The listing builds one solid part. Answer for the finished solid, in the listing's coordinates (mm). Round coordinates to 2 decimals unless told otherwise and drop trailing zeros. Write each loop counter-clockwise with the first axis right and the second up, starting at its lowest first coordinate (ties: lowest second). Pieces come first, ordered by that corner, then holes. Notation, with made-up numbers: M 43,-1.75 L 85,-1.75 A31 ccw 85,30.25 Z; hole C 29.5,-26 d2. An arc over 180 degrees is marked long. One line per item, written item: value. Start each with the question number.
(1) Section B-B (x = 0) is taken. Determine the outline of the cut face in (y, z), plus the area to 3 significant figures.
(2) Given P1, Ø8, axis at x = 68.5, y = 27, coming from the +Z side; P2, Ø3, axis at x = 14, y = 25.5, coming from the +Z side; P3, Ø5, axis at x = -91.5, y = 15, coming from the -Z side, each flat-ended and moving along its own axis, determine where each tip first touches the part or whether it passes through.
(3) Section D-D (x = -73.5) is taken. Determine the outline of the cut face in (y, z).
(4) Section A-A (z = 0) is taken. Determine the outline of the cut face in (x, y), plus the area to 3 significant figures.
(5) Section C-C (y = 24.25) is taken. Determine the outline of the cut face in (x, z).
(6) Consider probe 1 along Z at (x, y) = (0, 18.25); probe 2 along Z at (x, y) = (11.5, 26.75); probe 3 along Z at (x, y) = (0, 8.75). Determine where each line is inside the solid, lowest interval first.
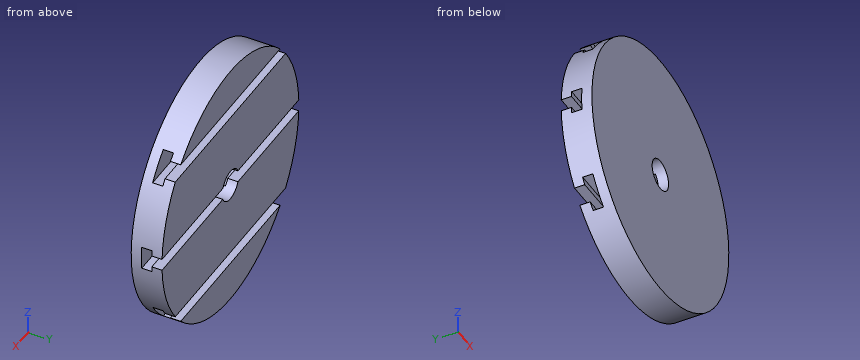
```python
from build123d import *

# Parameters (mm, degrees)
SKETCH_1_W          = 110
SKETCH_1_H          = 30
CUT_EXTRUDE_1_DEPTH = 150


with BuildPart() as part:
    # Эскиз1 → Повернуть1 (revolve)
    with BuildSketch(Plane(origin=(0, 0, 0), x_dir=(0, 0, -1), z_dir=(1, 0, 0))):
        with Locations((70, 15)):
            Rectangle(SKETCH_1_W, SKETCH_1_H)
    revolve(axis=Axis((0, -12.628115938, 0), (0, 1, 0)))

    # Эскиз2 → Вырез-Вытянуть1 (cut, symmetric)
    with BuildSketch(Plane(origin=(0, 0, 0), x_dir=(0, 0, -1), z_dir=(1, 0, 0))):
        Polygon((11.5, 10), (11.5, 20), (6, 20), (6, 30), (-6, 30), (-6, 20), (-11.5, 20), (-11.5, 10), align=None)
        Polygon((68.5, 10), (91.5, 10), (91.5, 20), (86, 20), (86, 30), (74, 30), (74, 20), (68.5, 20), align=None)
        Polygon((-91.5, 10), (-68.5, 10), (-68.5, 20), (-74, 20), (-74, 30), (-86, 30), (-86, 20), (-91.5, 20), align=None)
    extrude(amount=CUT_EXTRUDE_1_DEPTH, both=True, mode=Mode.SUBTRACT)


solid = part.part
```
Recorded:
1. outline: M 0,-125 L 30,-125 L 30,-86 L 20,-86 L 20,-91.5 L 10,-91.5 L 10,-68.5 L 20,-68.5 L 20,-74 L 30,-74 L 30,-15 L 0,-15 Z; M 0,15 L 30,15 L 30,74 L 20,74 L 20,68.5 L 10,68.5 L 10,91.5 L 20,91.5 L 20,86 L 30,86 L 30,125 L 0,125 Z
1. area: 5,900 mm2
2. P1: stops at z = 107.07
2. P2: stops at z = 124.37
2. P3: stops at z = -68.5
3. outline: M 0,-101.11 L 30,-101.11 L 30,-86 L 20,-86 L 20,-91.5 L 10,-91.5 L 10,-68.5 L 20,-68.5 L 20,-74 L 30,-74 L 30,-6 L 20,-6 L 20,-11.5 L 10,-11.5 L 10,11.5 L 20,11.5 L 20,6 L 30,6 L 30,74 L 20,74 L 20,68.5 L 10,68.5 L 10,91.5 L 20,91.5 L 20,86 L 30,86 L 30,101.11 L 0,101.11 Z
4. outline: M -125,0 L -15,0 L -15,10 L -125,10 Z; M 15,0 L 125,0 L 125,10 L 15,10 Z
4. area: 2,200 mm2
5. outline: M -124.86,-6 A125 ccw -100.74,-74 L 100.74,-74 A125 ccw 124.86,-6 L 13.75,-6 A15 cw -13.75,-6 Z; M -124.86,6 L -13.75,6 A15 cw 13.75,6 L 124.86,6 A125 ccw 100.74,74 L -100.74,74 A125 ccw Z; M -90.71,-86 A125 ccw 90.71,-86 Z; M -90.71,86 L 90.71,86 A125 ccw Z
6. probe 1: z = -125 to -91.5, -68.5 to -15, 15 to 68.5, 91.5 to 125
6. probe 2: z = -124.47 to -86, -74 to -9.63, 9.63 to 74, 86 to 124.47
6. probe 3: z = -125 to -15, 15 to 125
